```python
from build123d import *

# Parameters (mm, degrees)
SKETCH2_W           = 63.62
SKETCH2_H           = 39.62
SKETCH2_R           = 1.3208
SKETCH2_R_2         = 12.7
BOSS_EXTRUDE1_DEPTH = 2.54


with BuildPart() as part:
    # Sketch2 → Boss-Extrude1 (new body)
    with BuildSketch(Plane.XY):
        with Locations((0, -3.9477)):
            Rectangle(SKETCH2_W, SKETCH2_H)
        with Locations((-28, -19.9477)):
            Circle(SKETCH2_R, mode=Mode.SUBTRACT)
        with Locations((28, -19.9477)):
            Circle(SKETCH2_R, mode=Mode.SUBTRACT)
        with Locations((28, 12.0523)):
            Circle(SKETCH2_R, mode=Mode.SUBTRACT)
        with Locations((-28, 12.0523)):
            Circle(SKETCH2_R, mode=Mode.SUBTRACT)
        Circle(SKETCH2_R_2, mode=Mode.SUBTRACT)
    extrude(amount=BOSS_EXTRUDE1_DEPTH)


solid = part.part
```
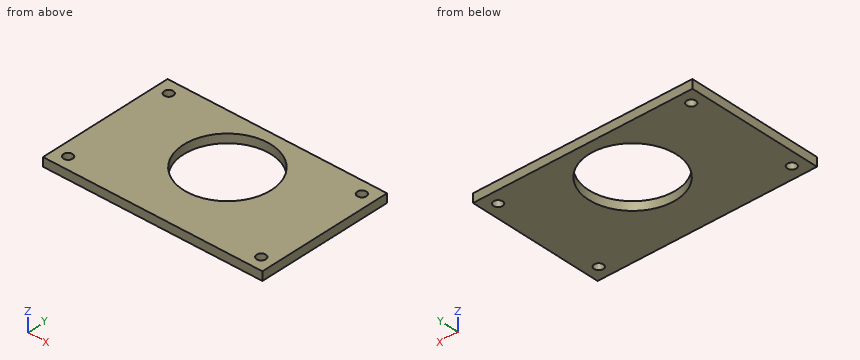
Check sheet for the modelled part. Datum: model origin and axes. Units: mm. Give positions to 0.01 mm unless a question says otherwise; leave off trailing zeros. Write each loop counter-clockwise with the first axis right and the second up, starting at its lowest first coordinate (ties: lowest second). Pieces come first, ordered by that corner, then holes. Notation, with made-up numbers: (41, 10) - (52, 10) arc R27 cw to (52, 42) - close; hole circle Ø11 at (41, 37). An arc over 180 degrees is marked (long way). Answer as a JSON object with one key per item and string values. Group by question number.
1) Sectioned sample at A-A (x = 0). Record the cut outline in (y, z).
2) Sectioned sample at C-C (y = 0). Record the cut outline in (x, z).
3) Thickness scan on probe 1 along Y at (x, z) = (-28, 1.65); probe 2 along Y at (x, z) = (27, 1.85); probe 3 along X at (y, z) = (11, 1.25). Record the ranges inside material, lowest first. Write a range as from..to.
4) Sectioned sample at D-D (z = 1.45). Record the cut outline in (x, y), then the cut area to 3 significant figures.
5) Sectioned sample at B-B (x = -28). Record the cut outline in (y, z), then the cut area to 3 significant figures.
Geometry results:
{
 "1": {"outline": "(-23.76, 0) - (-12.7, 0) - (-12.7, 2.54) - (-23.76, 2.54) - close; (12.7, 0) - (15.86, 0) - (15.86, 2.54) - (12.7, 2.54) - close"},
 "2": {"outline": "(-31.81, 0) - (-12.7, 0) - (-12.7, 2.54) - (-31.81, 2.54) - close; (12.7, 0) - (31.81, 0) - (31.81, 2.54) - (12.7, 2.54) - close"},
 "3": {"probe 1": "y = -23.76..-21.27, -18.63..10.73, 13.37..15.86", "probe 2": "y = -23.76..-20.81, -19.08..11.19, 12.92..15.86", "probe 3": "x = -31.81..-28.8, -27.2..-6.35, 6.35..27.2, 28.8..31.81"},
 "4": {"outline": "(-31.81, -23.76) - (31.81, -23.76) - (31.81, 15.86) - (-31.81, 15.86) - close; hole circle Ø2.64 at (-28, -19.95); hole circle Ø2.64 at (-28, 12.05); hole circle Ø25.4 at (0, 0); hole circle Ø2.64 at (28, -19.95); hole circle Ø2.64 at (28, 12.05)", "area": "1,990 mm^2"},
 "5": {"outline": "(-23.76, 0) - (-21.27, 0) - (-21.27, 2.54) - (-23.76, 2.54) - close; (-18.63, 0) - (10.73, 0) - (10.73, 2.54) - (-18.63, 2.54) - close; (13.37, 0) - (15.86, 0) - (15.86, 2.54) - (13.37, 2.54) - close", "area": "87.2 mm^2"}
}
